Verification items for this drawing (mm, ordinates from the low corner). A direction names the side the tool comes from. Give positions to 0.01 mm unless a question says otherwise; leave off trailing zeros. Loops run counter-clockwise (first coordinate to the right, second up) from the corner with the lowest first, then second, coordinate; pieces in that order, holes last. Notation, with made-up numbers: (-15.5, -30.5) -> (43.5, -30.5) arc R27 ccw to (43.5, -8.5) -> close; hole circle Ø6 at (30, 8). An arc over 180 degrees is marked (long way). Answer as CSV lines item,"result". Start each with the question number.
(1) Access from +Z, -Z, +X, -X, +Y, -Y to the whole of each face (thin tool, end or side, straight path). Record for the marked faces 1 and 2.
(2) Section check A-A on z = 16.01. Enter the section's corners in (x, y).
(3) Section check C-C on y = 65.5. Enter the section's corners in (x, z).
(4) Section check D-D on z = 9.5. Enter the section's corners in (x, y).
(5) Section check B-B on x = 15. Enter the section's corners in (y, z), plus the area to 3 significant figures.
(6) Material ranges on line 1 (X direction, y = 0.4, z = 16.01); line 2 (Z direction, x = 20, y = 35); line 3 (Y direction, x = 14.5, z = 16), recorded low to high. Write a range as from..to.
(7) Gauge pin test, flat end, axial feed: pin 1 Ø8 at (x, y) = (23.5, 54) entering from -Z. Record the tip position at first contact, or that the pin passes through.
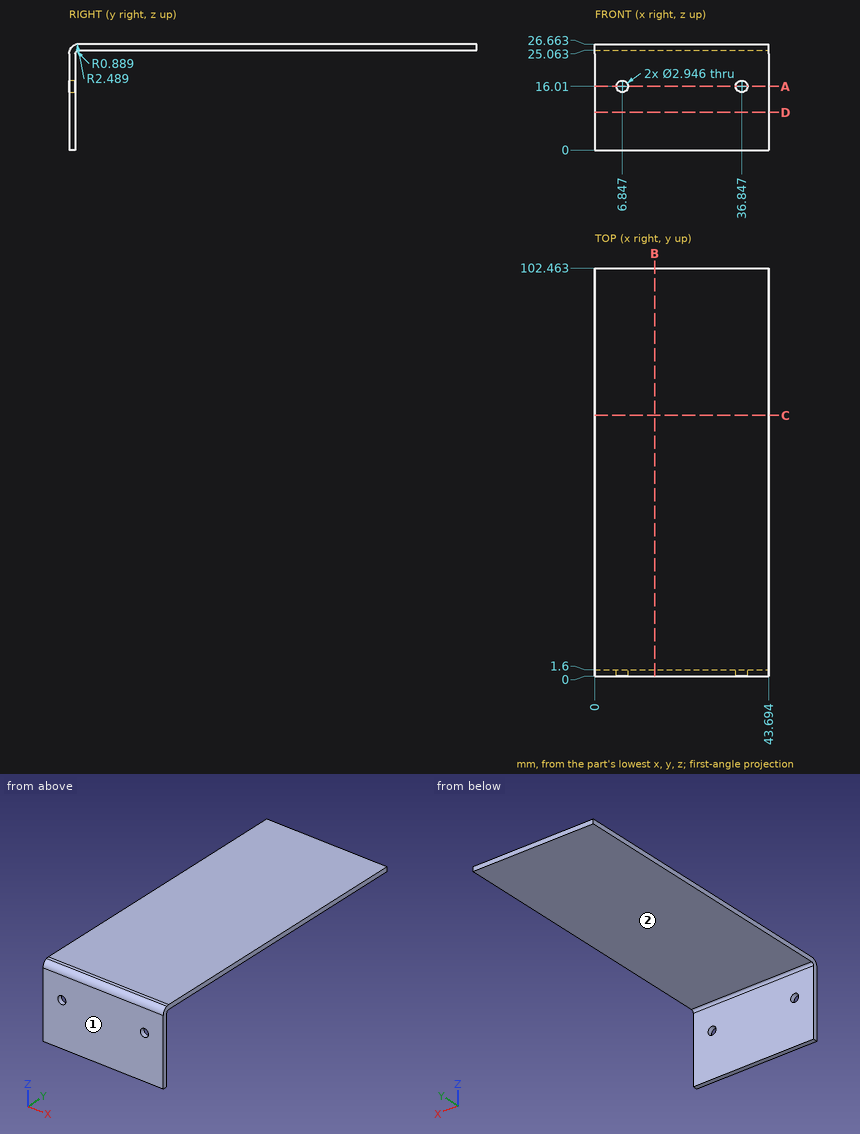
Working result:
1,face 1,"+Z, -Z, +X, -X, -Y"
1,face 2,"-Z, +X, -X, +Y"
2,outline,"(0, 0) -> (5.37, 0) -> (5.37, 1.6) -> (0, 1.6) -> close; (8.32, 0) -> (35.37, 0) -> (35.37, 1.6) -> (8.32, 1.6) -> close; (38.32, 0) -> (43.69, 0) -> (43.69, 1.6) -> (38.32, 1.6) -> close"
3,outline,"(0, 25.06) -> (43.69, 25.06) -> (43.69, 26.66) -> (0, 26.66) -> close"
4,outline,"(0, 0) -> (43.69, 0) -> (43.69, 1.6) -> (0, 1.6) -> close"
5,outline,"(0, 0) -> (1.6, 0) -> (1.6, 24.17) arc R0.89 cw to (2.49, 25.06) -> (102.46, 25.06) -> (102.46, 26.66) -> (2.49, 26.66) arc R2.49 ccw to (0, 24.17) -> close"
5,area,"203 mm^2"
6,line 1,"x = 0..5.37, 8.32..35.37, 38.32..43.69"
6,line 2,"z = 25.06..26.66"
6,line 3,"y = 0..1.6"
7,pin 1,"stops at z = 25.06"
